Input: part model. Units: mm. Frame: model coordinates. Face numbers are marked on the shaded views. Coordinates: 2 decimals unless noted, no trailing zeros. Loops run counter-clockwise (first coordinate to the right, second up) from the corner with the lowest first, then second, coordinate; pieces in that order, holes last. Notation, with made-up numbers: M -9.75,-32 L 11.25,-32 A25 cw 11.25,-5 Z; hole C 49,-8.75 d10. An arc over 180 degrees is marked long. Use a Markdown table: item, result. Add a question column.
1. Section B-B on y = 12.5. Output: boundary loops of the cut face in (x, z), then the cut area to 3 significant figures.
2. Line query: L1, parallel to Y at x = 2.5, z = 2.2; L2, parallel to X at y = 13.75, z = 1.3. Output: solid intervals per line, ascending. Write a range as [from, to].
3. Section C-C on z = 0.6. Output: boundary loops of the cut face in (x, y).
4. Section A-A on x = 2.5. Output: boundary loops of the cut face in (y, z), then the cut area to 3 significant figures.
5. Draft query along X for the marked faces 1, 2, 3 and 4. Return one class per face: +X half, -X half, draft (parallel to the pull), parting line (faces both ways), or undercut.
```python
from build123d import *

# Parameters (mm, degrees)
F1_W     = 5
F1_H     = 25
F2_DEPTH = 5
F3_R     = 1.5
F4_DEPTH = 5.001


with BuildPart() as f2:
    # F1 (on Top) → F2 (new body)
    with BuildSketch(Plane.XY):
        with Locations((2.5, 12.5)):
            Rectangle(F1_W, F1_H)
    extrude(amount=F2_DEPTH)

    # F3 (on face) → F4 (cut, through all)
    with BuildSketch(Plane.XY.offset(5)):
        with Locations((2.5, 12.5)):
            Circle(F3_R)
        with BuildLine():
            Line((1, 0), (4, 0))
            ThreePointArc((4, 0), (2.5, 1.5), (1, 0))
        make_face()
        with BuildLine():
            ThreePointArc((1, 25), (2.5, 23.5), (4, 25))
            Line((4, 25), (1, 25))
        make_face()
    extrude(amount=-F4_DEPTH, mode=Mode.SUBTRACT)


solid = f2.part
```
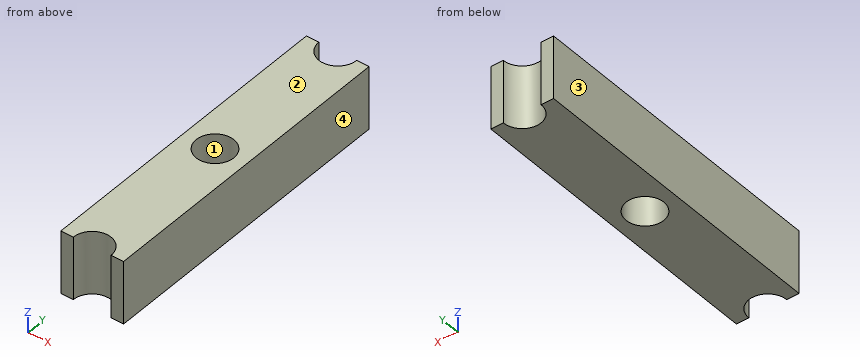
Answers below:
| question | item | result |
|---|---|---|
| 1 | outline | M 0,0 L 1,0 L 1,5 L 0,5 Z; M 4,0 L 5,0 L 5,5 L 4,5 Z |
| 1 | area | 10.0 mm² |
| 2 | L1 | y = [1.5, 11], [14, 23.5] |
| 2 | L2 | x = [0, 1.67], [3.33, 5] |
| 3 | outline | M 0,0 L 1,0 A1.5 cw 4,0 L 5,0 L 5,25 L 4,25 A1.5 cw 1,25 L 0,25 Z; hole C 2.5,12.5 d3 |
| 4 | outline | M 1.5,0 L 11,0 L 11,5 L 1.5,5 Z; M 14,0 L 23.5,0 L 23.5,5 L 14,5 Z |
| 4 | area | 95.0 mm² |
| 5 | face 1 | undercut |
| 5 | face 2 | draft |
| 5 | face 3 | -X half |
| 5 | face 4 | +X half |
